Could you check a few things on this model? Use its own coordinates, in mm. Face numbers are marked on the shaded views. A direction names the side the tool comes from. Round coordinates to 2 decimals unless told otherwise and drop trailing zeros. Order: outer loops, then holes, each group sorted by start corner. A loop starts at its lowest first (then second) coordinate and runs counter-clockwise, first axis right, second up. Notation, with made-up numbers: (15.5, 62) -> (69.5, 62) arc R16 ccw to (69.5, 76) -> close; hole circle Ø4 at (-22, 63). An arc over 180 degrees is marked (long way). Put each result on its own line as item: value. Start each with the question number.
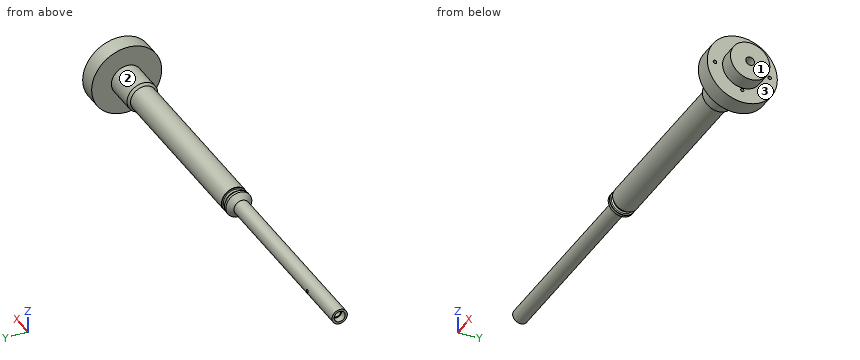
Autodesk Inventor part; units mm, degrees
ref_plane "YZ Plane" through (0, 0, 0) normal (1, 0, 0) x (0, 1, 0)
ref_plane "XZ Plane" through (0, 0, 0) normal (0, 1, 0) x (-1, 0, 0)
ref_plane "XY Plane" through (0, 0, 0) normal (0, 0, 1) x (1, 0, 0)
sketch "Skizze1" plane through (0, 0, 0) normal (0, 0, 1) x (1, 0, 0)
  line L0 (-0.0085, 0) -> (-0.0085, 9)
  line L1 (-7.0085, 16) -> (-15.0085, 16)
  line L2 (-15.0085, 16) -> (-15.0085, 7)
  line L3 (-30.0085, 5.925) -> (-111.1085, 5.925)
  line L4 (-113.8085, 5.925) -> (-115.0085, 5.925)
  line L5 (-115.0085, 5.925) -> (-117.4335, 3.5)
  line L6 (-117.4335, 3.5) -> (-204.9135, 3.5)
  line L7 (-204.9135, 3.5) -> (-204.9135, 0)
  line L8 (-222.883, 3.2454) -> (-222.883, 3.2454)
  line L9 (-222.883, 3.2454) -> (-222.883, 3.2454)
  line L10 (-204.9135, 0) -> (-0.0085, 0)
  line L11 (-111.8085, 4.5) -> (-113.1085, 4.5)
  line L12 (-30.0085, 5.925) -> (-29.0085, 7)
  line L13 (-29.0085, 7) -> (-15.0085, 7)
  line L14 (-113.7085, 5.1) -> (-113.7085, 5.825)
  line L15 (-111.2085, 5.1) -> (-111.2085, 5.825)
  arc A0 (-113.7085, 5.1) -> (-113.1085, 4.5) centre (-113.1085, 5.1) ccw
  arc A1 (-111.8085, 4.5) -> (-111.2085, 5.1) centre (-111.8085, 5.1) ccw
  arc A2 (-111.1085, 5.925) -> (-111.2085, 5.825) centre (-111.1085, 5.825) ccw
  arc A3 (-113.7085, 5.825) -> (-113.8085, 5.925) centre (-113.8085, 5.825) ccw
  line L16 (-7.0085, 16) -> (-7.0085, 9)
  line L17 (-7.0085, 9) -> (-0.0085, 9)
  point P0 (-111.2085, 5.925)
  point P1 (-113.7085, 5.925)
  point P2 (-111.2085, 4.5)
  point P3 (-113.7085, 4.5)
  dimension "d19" = 14
  dimension "d20" = 15
  dimension "d21" = 7
  dimension "d22" = 5.925
  dimension "d23" = 4.5
  dimension "d24" = 3.5
  dimension "d26" = 47.07
  dimension "d27" = 45
  dimension "d33" = 2.5
  dimension "d34" = 1.3
  dimension "d35" = 87.48
  dimension "d44" = 0.6
  dimension "d45" = 0.1
  dimension "d127" = 16
  dimension "d128" = 8
  dimension "d129" = 7
  dimension "d130" = 9
  dimension "d152" = 189.905
  dimension "d153" = 174.905
  dimension "d154" = 111.2
  dimension "d156" = 81.2
  dimension "d157" = 2.425
revolve "Drehung2" add sketch "Skizze1" angle 360 about axis through (-204.9135, 0, 0) along (1, 0, 0)
ref_plane "Arbeitsebene1" through (-161.1735, 3.5, 0) normal (0, 1, 0) x (-1, 0, 0)
sketch "Skizze3" plane through (-161.1735, 3.5, 0) normal (0, 1, 0) x (-1, 0, 0)
  line L0 (-43.74, 3.5) -> (-43.74, -3.5)
  line L1 (43.74, 3.5) -> (43.74, -3.5)
  line L2 (43.74, 3.5) -> (-43.74, 3.5)
  line L3 (43.74, -3.5) -> (-43.74, -3.5)
  line L4 (-222.6365, 0) -> (64.2305, 0)
  point P0 (21.74, 0)
  dimension "d158" = 65.48
  dimension "d166" = 22
hole "Bohrung1" at (-182.9135, 3.5, 0) direction (0, -1, 0) diameter 1.5 depth 3.5
hole "Bohrung2" at (-0.0085, 0, 0) direction (-1, 0, 0) diameter 4 depth 223
sketch "Skizze4" plane through (-15.0085, 0, 0) normal (-1, 0, 0) x (0, 0, 1)
  circle A0 centre (0, 0) radius 16
  circle A1 centre (0, 0) radius 16
  circle A2 centre (0, 0) radius 7
  circle A3 centre (0, 0) radius 7
  line L0 (0, -19.2) -> (0, 25.6)
  circle A4 centre (0, 0) radius 9
  point P0 (-10, 0)
  point P1 (0, 11.7051)
  dimension "d132" = 90
  dimension "d148" = 10
hole "Bohrung3" at (-15.0085, 0, -10) direction (1, 0, 0) diameter 1.5 depth 8
sketch "Skizze17" plane through (-7.0085, 0, 0) normal (1, 0, 0) x (0, 0, -1)
  circle A0 centre (0, 0) radius 16
  line L0 (0, -19.2) -> (0, 25.6)
  circle A1 centre (0, 0) radius 9
  point P0 (0, 12.5)
  point P1 (0, -12.5)
  point P2 (0, 9)
  point P3 (0, 16)
  point P4 (0, -16)
  point P5 (0, -9)
  dimension "d135" = 7
  dimension "d136" = 3.5
  dimension "d137" = 3.5
  dimension "d145" = 12.5
hole "Bohrung10" at (-7.0085, -12.5, 0) at (-7.0085, 12.5, 0) direction (-1, 0, 0) diameter 1.567 depth 6 tip angle 118
sketch "Skizze19" plane through (-204.9135, 0, 0) normal (-1, 0, 0) x (0, 0, 1)
  circle A0 centre (0, 0) radius 2
hole "Bohrung11" at (-204.9135, 0, 0) direction (1, 0, 0) diameter 5 depth 3
properties part number "Halter02"
1. For pin 1 Ø4 at (y, z) = (-4, -7.5) entering from -X; pin 2 Ø10 at (y, z) = (-1, -4) entering from -X; pin 3 Ø10 at (x, z) = (-34, -3.5) entering from +Y; pin 4 Ø6 at (x, y) = (-53, 5) entering from -Z, each with a flat end and sliding along its axis, tell me the tip position at first contact or that it passes through.
2. I need wall thicknesses on L1, parallel to Z at x = -9, y = 0; L2, parallel to Z at x = -108.5, y = 0 (3 decimals); L3, parallel to Z at x = -204, y = 0. Which ranges of each line are inside material? Lowest first, please.
3. If we section it at B-B, the plane x = -62.5: Please give me the cut outline in (y, z) (3 decimals).
4. Which directions (+Z, -Z, +X, -X, +Y, -Y) give clear straight access to the entire face, cutting with the end or side of a thin tool? Please do the marked faces 1, 2 and 3.
5. If we section it at A-A, the plane x = -161.5: Please give me the cut outline in (y, z), then the cut area to 3 significant figures.
Results below:
1. pin 1: x = -29.47
1. pin 2: x = -204.91
1. pin 3: y = 6.46
1. pin 4: z = -5.58
2. L1: -16 to -10.75, -9.25 to -2, 2 to 16
2. L2: -5.925 to -2, 2 to 5.925
2. L3: -3.5 to -2.5, 2.5 to 3.5
3. outline: circle Ø11.85 at (0, 0); hole circle Ø4 at (0, 0)
4. face 1: +Z, -Z, +X, +Y, -Y
4. face 2: -X
4. face 3: +X
5. outline: circle Ø7 at (0, 0); hole circle Ø4 at (0, 0)
5. area: 25.9 mm2
